Source: three-view drawing plus pictorial views. Frame: mm from the lowest corner of the part. A direction names the side the tool comes from. Give positions to 0.01 mm unless a question says otherwise; leave off trailing zeros. Order: outer loops, then holes, each group sorted by start corner. A loop starts at its lowest first (then second) coordinate and runs counter-clockwise, first axis right, second up. Notation, with made-up numbers: (35.25, 23) -> (91.25, 23) arc R26 ccw to (91.25, 39) -> close; hole circle Ø4 at (72, 71.5). An arc over 180 degrees is marked (long way). One line per question, with ' | ' between items.
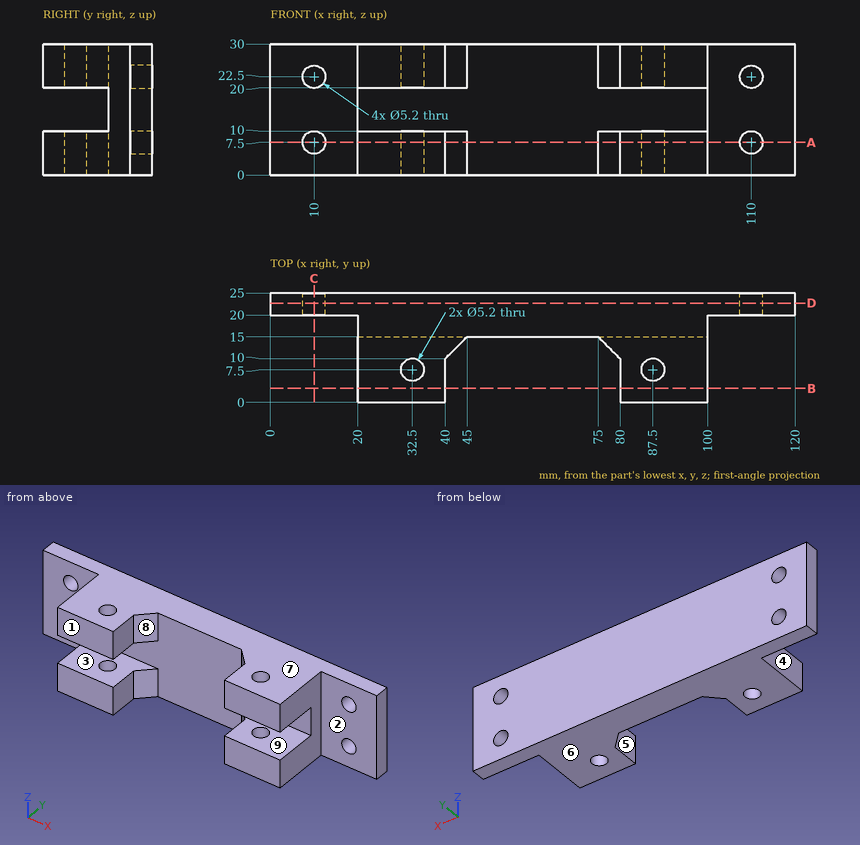
1) Section C-C on x = 10. Return loops of the section in (y, z), plus the area to 3 significant figures.
Check result:
outline: (20, 0) -> (25, 0) -> (25, 4.9) -> (20, 4.9) -> close; (20, 10.1) -> (25, 10.1) -> (25, 19.9) -> (20, 19.9) -> close; (20, 25.1) -> (25, 25.1) -> (25, 30) -> (20, 30) -> close | area: 98.0 mm^2
2) Section D-D on y = 22.75. Return loops of the section in (x, z).
Check result:
outline: (0, 0) -> (120, 0) -> (120, 30) -> (0, 30) -> close; hole circle Ø5.2 at (10, 7.5); hole circle Ø5.2 at (10, 22.5); hole circle Ø5.2 at (110, 7.5); hole circle Ø5.2 at (110, 22.5)
3) Set-up query: the marked faces 1, 2, 3, 4 and 5. Return all of +Z, -Z, +X, -X, +Y, -Y with unobstructed straight access to the full face (end or side cutting, diameter ignored); none if empty.
Check result:
face 1: +Z, -Z, +X, -X, -Y | face 2: +Z, -Z, +X, -Y | face 3: +X, -X, -Y | face 4: +Z, -Z, -X, -Y | face 5: +Z, -Z, -Y
4) Material intervals for probe 1 along X at (y, z) = (21.5, 22.25); probe 2 along Y at (x, z) = (32.5, 27.5); probe 3 along Z at (x, y) = (97, 1.5), sorted ascending. Write a range as from..to.
Check result:
probe 1: x = 0..7.41, 12.59..107.41, 112.59..120 | probe 2: y = 0..4.9, 10.1..25 | probe 3: z = 0..10, 20..30
5) Contact query for flat-ended pins moving along their axis: pin 1 Ø12 at (y, z) = (5, 5) entering from -X; pin 2 Ø11 at (y, z) = (4, 3) entering from +X; pin 3 Ø9 at (x, z) = (64, 15) entering from -Y. Output: stop coordinate, or through.
Check result:
pin 1: stops at x = 20 | pin 2: stops at x = 100 | pin 3: stops at y = 15
6) Pull-direction query (Z, two-part tool) for the marked faces 6, 7, 8 and 9; classes: +Z half, -Z half, draft (parallel to the pull), parting line (faces both ways), or undercut.
Check result:
face 6: -Z half | face 7: +Z half | face 8: draft | face 9: undercut
7) Section B-B on y = 3.25. Return loops of the section in (x, z).
Check result:
outline: (20, 0) -> (40, 0) -> (40, 10) -> (20, 10) -> close; (20, 20) -> (40, 20) -> (40, 30) -> (20, 30) -> close; (80, 0) -> (100, 0) -> (100, 10) -> (80, 10) -> close; (80, 20) -> (100, 20) -> (100, 30) -> (80, 30) -> close
8) Section A-A on z = 7.5. Return loops of the section in (x, y).
Check result:
outline: (0, 20) -> (7.4, 20) -> (7.4, 25) -> (0, 25) -> close; (12.6, 20) -> (20, 20) -> (20, 0) -> (40, 0) -> (40, 10) -> (45, 15) -> (75, 15) -> (80, 10) -> (80, 0) -> (100, 0) -> (100, 20) -> (107.4, 20) -> (107.4, 25) -> (12.6, 25) -> close; (112.6, 20) -> (120, 20) -> (120, 25) -> (112.6, 25) -> close; hole circle Ø5.2 at (32.5, 7.5); hole circle Ø5.2 at (87.5, 7.5)
